Could you check a few things on this drawing? It's one solid part, dimensions in mm from its lowest x, y, z. Coordinates: 2 decimals unless noted, no trailing zeros. Write each loop counter-clockwise with the first axis right and the second up, starting at its lowest first coordinate (ties: lowest second). Pieces come first, ordered by that corner, then holes. Notation, with made-up numbers: M 4,13 L 36,13 A16 ccw 36,41 Z; hole C 49.5,86.5 d5. An arc over 180 degrees is marked long. Use a Markdown table: item, result.
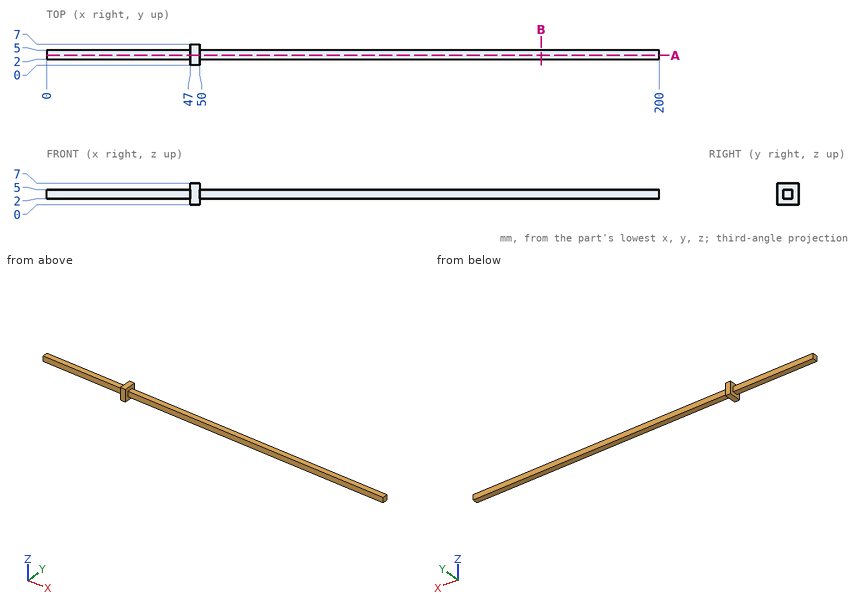
1. Suppose I cut it at A-A on y = 3.25. Write out the boundary of the cut face in (x, z).
Answers follow:
| item | result |
|---|---|
| outline | M 0,2 L 47,2 L 47,0 L 50,0 L 50,2 L 200,2 L 200,5 L 50,5 L 50,7 L 47,7 L 47,5 L 0,5 Z |
2. Suppose I cut it at B-B on x = 161.5. Write out the boundary of the cut face in (y, z).
Answers follow:
| item | result |
|---|---|
| outline | M 2,2 L 5,2 L 5,5 L 2,5 Z |
3. Will these pins go through, and if not, where does the flat tip stop? pin 1 Ø1.5 at (x, y) = (110, 3) entering from +Z; pin 2 Ø3.5 at (x, z) = (23.5, 3.5) entering from +Y; pin 3 Ø2 at (x, z) = (100, 1.5) entering from -Y; pin 4 Ø3 at (y, z) = (1.5, 3) entering from +X.
Answers follow:
| item | result |
|---|---|
| pin 1 | stops at z = 5 |
| pin 2 | stops at y = 5 |
| pin 3 | stops at y = 2 |
| pin 4 | stops at x = 200 |
4. I need wall thicknesses on probe 1 along Y at (x, z) = (127, 4.75); probe 2 along X at (y, z) = (2, 6.5). Which ranges of each line are inside material? Lowest first, please.
Answers follow:
| item | result |
|---|---|
| probe 1 | y = 2 to 5 |
| probe 2 | x = 47 to 50 |
